The model under review builds one solid part; all positions refer to its coordinate system, in mm. Face numbers are marked on the shaded views. A direction names the side the tool comes from. Coordinates: 2 decimals unless noted, no trailing zeros. Order: outer loops, then holes, each group sorted by start corner. A loop starts at its lowest first (then second) coordinate and runs counter-clockwise, first axis right, second up. Notation, with made-up numbers: M -11,-4.75 L -5,-4.75 A18 ccw -5,30.25 Z; hole C 30.5,72.25 d10. An arc over 180 degrees is marked long. Answer as CSV lines item,"result". Start each with the question number.
Q1. Consider section B-B on x = 5.5. Write out the cut boundary in (y, z), and give its area (3 significant figures).
Q2. For P1, Ø5, axis at y = 33, z = 5, coming from the +X side; P2, Ø4, axis at x = 14, z = 5, coming from the +Y side; P3, Ø6, axis at x = 7.5, z = 8, coming from the -Y side, all flat-tipped, find the tip position at first contact; note any pin that passes through.
Q3. The part is to be moulded in two halves that separate along Y. For the marked faces 6, 7, 8 and 9, say which applies: +Y half, -Y half, draft (parallel to the pull), parting line (faces both ways), or undercut.
Q4. Consider section C-C on z = 5. Write out the cut boundary in (x, y).
Q5. Machinability: for the marked faces 1, 2, 3, 4 and 5, which of the approach directions +Z, -Z, +X, -X, +Y, -Y give a long, thin tool a straight path to every point of the face, cutting with its end or side? Answer none if there is none.
Q6. Consider section D-D on y = 11. Write out the cut boundary in (x, z), and give its area (3 significant figures).
Q7. Consider section A-A on y = -9. Write out the cut boundary in (x, z), and give its area (3 significant figures).
Q8. Wall thickness on L1, parallel to Y at x = 20, z = 6.75; L2, parallel to Y at x = 1.05, z = 5; L3, parallel to Y at x = 1.3, z = 5: over which ranges is each line inside the solid? List them lowest first. Write a range as [from, to].
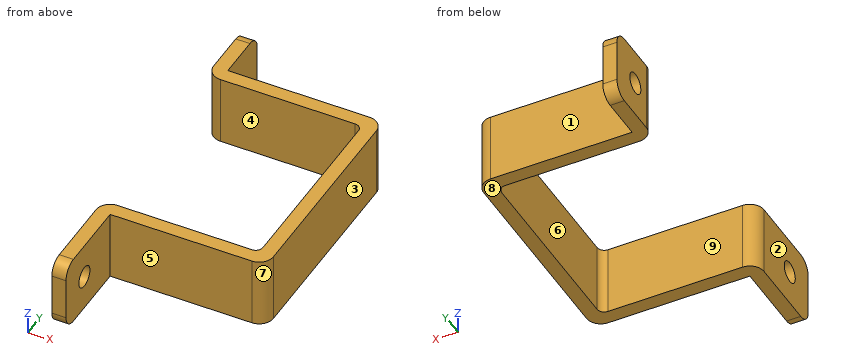
Autodesk Inventor part; units mm, degrees
ref_plane "YZ Plane" through (0, 0, 0) normal (1, 0, 0) x (0, 1, 0)
ref_plane "XZ Plane" through (0, 0, 0) normal (0, 1, 0) x (-1, 0, 0)
ref_plane "XY Plane" through (0, 0, 0) normal (0, 0, 1) x (1, 0, 0)
sketch "Skizze1" plane through (0, 0, 0) normal (0, 0, 1) x (1, 0, 0)
  line L0 (0, 0) -> (22, 0)
  line L1 (22, 0) -> (22, 28)
  line L2 (22, 28) -> (0, 28)
  line L3 (0, 28) -> (0, 38)
  line L4 (0, 38) -> (2, 38)
  line L5 (2, 38) -> (2, 30)
  line L6 (2, 30) -> (24, 30)
  line L7 (24, 30) -> (24, -2)
  line L8 (24, -2) -> (2, -2)
  line L9 (2, -2) -> (2, -14)
  line L10 (2, -14) -> (0, -14)
  line L11 (0, -14) -> (0, 0)
  line L12 (22, 0) -> (22, -2) construction
  line L13 (22, 28) -> (22, 30) construction
  dimension "d1" = 14
  dimension "d3" = 2
  dimension "d4" = 20
  dimension "d5" = 2
  dimension "d6" = 28
  dimension "d7" = 2
  dimension "d17" = 10
extrude "Extrusion1" add sketch "Skizze1" along normal blind 10
fillet "Rundung1" radius 2 4 edges at (0, 28, 5) (0, 0, 5) (24, 30, 5) (24, -2, 5)
fillet "Rundung2" radius 2 4 edges at (1, -14, 10) (1, -14, 0) (1, 38, 10) (1, 38, 0)
sketch "Skizze2" plane through (0, 30, 0) normal (-1, 0, 0) x (0, 0, 1)
  line L0 (2, 8) -> (8, 8) construction
  line L1 (5, 8) -> (5, -2) construction
  line L2 (0, -2) -> (10, -2) construction
  circle A0 centre (5, 3) radius 1.5
  line L3 (10, -2) -> (10, -30) construction
  line L4 (0, -2) -> (0, -30) construction
  circle A1 centre (5, -39) radius 1.5
  line L5 (0, -32) -> (10, -32)
  point P0 (10, -4)
  point P1 (10, -28)
  point P2 (0, -4)
  point P3 (0, -28)
  point P4 (0, 0)
  dimension "d12" = 3
  dimension "d15" = 3
  dimension "d18" = 7
extrude "Extrusion2" cut sketch "Skizze2" against normal up to next
fillet "Rundung3" radius 1 2 edges at (22, 28, 5) (22, 0, 5)
properties part number "Akkuhalterung" material "ABS-Kunststoff"
Evaluation:
1,outline,"M -2,0 L 0,0 L 0,10 L -2,10 Z; M 28,0 L 30,0 L 30,10 L 28,10 Z"
1,area,"40.0 mm²"
2,P1,"stops at x = 2"
2,P2,"stops at y = 30"
2,P3,"stops at y = -2"
3,face 6,"undercut"
3,face 7,"-Y half"
3,face 8,"draft"
3,face 9,"undercut"
4,outline,"M 0,-14 L 2,-14 L 2,-10.5 L 0,-10.5 Z; M 0,-7.5 L 2,-7.5 L 2,-2 L 22,-2 A2 ccw 24,0 L 24,28 A2 ccw 22,30 L 2,30 L 2,31.5 L 0,31.5 L 0,30 A2 ccw 2,28 L 21,28 A1 cw 22,27 L 22,1 A1 cw 21,0 L 2,0 A2 ccw 0,-2 Z; M 0,34.5 L 2,34.5 L 2,38 L 0,38 Z"
5,face 1,"+Z, -Z, +X, +Y"
5,face 2,"+Z, -Z, -X, +Y, -Y"
5,face 3,"+Z, -Z, +X, +Y, -Y"
5,face 4,"+Z, -Z, -X"
5,face 5,"+Z, -Z, +X, -Y"
6,outline,"M 22,0 L 24,0 L 24,10 L 22,10 Z"
6,area,"20.0 mm²"
7,outline,"M 0,0 L 2,0 L 2,3.5 L 0,3.5 Z; M 0,6.5 L 2,6.5 L 2,10 L 0,10 Z"
7,area,"14.0 mm²"
8,L1,"y = [-2, 0], [28, 30]"
8,L2,"y = [-14, -10.5], [-7.5, -0.24], [28.24, 31.5], [34.5, 38]"
8,L3,"y = [-14, -10.5], [-7.5, -0.13], [28.13, 31.5], [34.5, 38]"
